Verification items for the finished model (mm, model axes). A direction names the side the tool comes from. Round coordinates to 2 decimals unless told otherwise and drop trailing zeros. Write each loop counter-clockwise with the first axis right and the second up, starting at its lowest first coordinate (ties: lowest second). Pieces come first, ordered by that corner, then holes. Notation, with made-up numbers: (22, -7) - (45, -7) arc R20 cw to (45, 24) - close; hole circle Ø6 at (1, -13.75). An arc over 180 degrees is marked (long way). Write each question's results on one line, items separated by ' | '.
```python
from build123d import *

# Parameters (mm, degrees)
BOSS_EXTRUDE1_DEPTH = 8
CUT_EXTRUDE1_DEPTH  = 2
SKETCH4_R           = 2
CUT_EXTRUDE2_DEPTH  = 2
SKETCH5_R           = 1
CUT_EXTRUDE3_DEPTH  = 22
CUT_EXTRUDE4_DEPTH  = 3


with BuildPart() as part:
    # Sketch1 → Boss-Extrude1 (new body)
    with BuildSketch(Plane.XY):
        with BuildLine():
            Line((8.5, 4), (8.5, 5))
            Line((8.5, 5), (-8.5, 5))
            Line((-8.5, 5), (-8.5, 4))
            Line((-8.5, 4), (-7.5, 4))
            Line((-7.5, 4), (-7.5, 1))
            Line((-7.5, 1), (-3.5, 1))
            ThreePointArc((-3.5, 1), (-2.5, 0), (-3.5, -1))
            Line((-3.5, -1), (-7.5, -1))
            Line((-7.5, -1), (-7.5, -4))
            Line((-7.5, -4), (-8.5, -4))
            Line((-8.5, -4), (-8.5, -5))
            Line((-8.5, -5), (8.5, -5))
            Line((8.5, -5), (8.5, -4))
            Line((8.5, -4), (7.5, -4))
            Line((7.5, -4), (7.5, 4))
            Line((7.5, 4), (8.5, 4))
        make_face()
    extrude(amount=BOSS_EXTRUDE1_DEPTH)

    # Sketch3 → Cut-Extrude1 (cut)
    with BuildSketch(Plane.XY.offset(8)):
        with BuildLine():
            Line((0.5, 4), (0.5, 5))
            Line((0.5, 5), (-8.5, 5))
            Line((-8.5, 5), (-8.5, 4))
            Line((-8.5, 4), (-7.5, 4))
            Line((-7.5, 4), (-7.5, 1))
            Line((-7.5, 1), (-3.5, 1))
            ThreePointArc((-3.5, 1), (-2.5, 0), (-3.5, -1))
            Line((-3.5, -1), (-7.5, -1))
            Line((-7.5, -1), (-7.5, -4))
            Line((-7.5, -4), (-8.5, -4))
            Line((-8.5, -4), (-8.5, -5))
            Line((-8.5, -5), (0.5, -5))
            Line((0.5, -5), (0.5, -4))
            Line((0.5, -4), (3.5, -3))
            Line((3.5, -3), (7.5, -3))
            Line((7.5, -3), (7.5, 3))
            Line((7.5, 3), (3.5, 3))
            Line((3.5, 3), (0.5, 4))
        make_face()
    extrude(amount=-CUT_EXTRUDE1_DEPTH, mode=Mode.SUBTRACT)

    # Sketch4 → Cut-Extrude2 (cut)
    with BuildSketch(Plane.XY.offset(6)):
        with Locations((4.062000401, 0)):
            Circle(SKETCH4_R)
    extrude(amount=-CUT_EXTRUDE2_DEPTH, mode=Mode.SUBTRACT)

    # Sketch5 → Cut-Extrude3 (cut)
    with BuildSketch(Plane.XY.offset(4)):
        with Locations((4.062000401, 0)):
            Circle(SKETCH5_R)
    extrude(amount=-CUT_EXTRUDE3_DEPTH, mode=Mode.SUBTRACT)

    # Sketch6 → Cut-Extrude4 (cut)
    with BuildSketch(Plane.XY.offset(6)):
        with BuildLine():
            Line((-6.5, 3), (-6.5, 4))
            Line((-6.5, 4), (-7.5, 4))
            Line((-7.5, 4), (-7.5, -4))
            Line((-7.5, -4), (-6.5, -4))
            Line((-6.5, -4), (-6.5, -3))
            Line((-6.5, -3), (-3.5, -3))
            ThreePointArc((-3.5, -3), (-0.5, 0), (-3.5, 3))
            Line((-3.5, 3), (-6.5, 3))
        make_face()
    extrude(amount=-CUT_EXTRUDE4_DEPTH, mode=Mode.SUBTRACT)


solid = part.part
```
(1) Section check C-C (z = 7). Record the cut outline in (x, y), plus the area to 3 significant figures.
Answer:
outline: (0.5, -5) - (8.5, -5) - (8.5, -4) - (7.5, -4) - (7.5, -3) - (3.5, -3) - (0.5, -4) - close; (0.5, 4) - (3.5, 3) - (7.5, 3) - (7.5, 4) - (8.5, 4) - (8.5, 5) - (0.5, 5) - close | area: 27.0 mm2
(2) Section check B-B (x = -4.25). Record the cut outline in (y, z).
Answer:
outline: (-5, 0) - (-1, 0) - (-1, 3) - (-3, 3) - (-3, 6) - (-5, 6) - close; (1, 0) - (5, 0) - (5, 6) - (3, 6) - (3, 3) - (1, 3) - close
(3) Mould release check, pull along X, two halves, no side actions. Record for faces 4 (the flat face through (-2, 0, 3)), 5 (the flat face through (5, -1, 4)), 6 (the flat face through (-8.5, 4.5, 3)): released by +X, released by -X, zero draft, split by the parting line, or undercut.
Answer:
face 4: zero draft | face 5: undercut | face 6: released by -X
(4) Thickness scan on L1, parallel to Y at x = 6.5, z = 7.25; L2, parallel to Z at x = -0.5, y = 1.25; L3, parallel to Z at x = 5.25, y = 0.5. Record the ranges inside material, lowest first.
Answer:
L1: -5 to -3, 3 to 5 | L2: 0 to 6 | L3: 0 to 4
(5) Set-up check for faces 1 (the flat face through (-6.5, -3.5, 4.5)), 2 (the flat face through (0.5, 4.5, 7)), 3 (the flat face through (-6, 1, 1)): record each of +Z, -Z, +X, -X, +Y, -Y from which the full face is reachable in a straight line by a thin tool's end or side.
Answer:
face 1: +Z, -X | face 2: +Z, -X, +Y, -Y | face 3: +Z, -Z, -X
(6) Go/stop test with flat-tipped pins: pin 1 Ø0.5 at (y, z) = (3.5, 5) entering from -X; pin 2 Ø3 at (x, y) = (-2.5, -0.5) entering from +Z; pin 3 Ø2 at (y, z) = (-2, 1.5) entering from +X. Record where each tip stops, or that it passes through.
Answer:
pin 1: x = -6.5 | pin 2: z = 3 | pin 3: x = 7.5
(7) Section check D-D (z = 1.5). Record the cut outline in (x, y).
Answer:
outline: (-8.5, -5) - (8.5, -5) - (8.5, -4) - (7.5, -4) - (7.5, 4) - (8.5, 4) - (8.5, 5) - (-8.5, 5) - (-8.5, 4) - (-7.5, 4) - (-7.5, 1) - (-3.5, 1) arc R1 cw to (-3.5, -1) - (-7.5, -1) - (-7.5, -4) - (-8.5, -4) - close; hole circle Ø2 at (4.06, 0)
(8) Section check A-A (y = 0). Record the cut outline in (x, z), plus the area to 3 significant figures.
Answer:
outline: (-2.5, 0) - (3.06, 0) - (3.06, 4) - (2.06, 4) - (2.06, 6) - (-0.5, 6) - (-0.5, 3) - (-2.5, 3) - close; (5.06, 0) - (7.5, 0) - (7.5, 6) - (6.06, 6) - (6.06, 4) - (5.06, 4) - close | area: 38.0 mm2
